from build123d import *

# Parameters (mm, degrees)
F1_DEPTH = 0.43
F2_R     = 0.114538
F2_R_2   = 0.135459
F3_DEPTH = 25
F4_W     = 0.697841
F4_H     = 0.5
F4_W_2   = 0.446198
F4_H_2   = 0.226708
F5_DEPTH = 0.13
F7_DEPTH = 25
F8_W     = 0.044617
F8_H     = 0.11
F8_W_2   = 0.05577
F8_W_3   = 0.03778
F8_W_4   = 0.051917
F9_DEPTH = 0.03


with BuildPart() as f1:
    # F0 (on Top) → F1 (new body)
    with BuildSketch(Plane.XY):
        with BuildLine():
            Line((-17.317478, 8.504073), (-17.317478, 21.504073))
            Line((-17.317478, 21.504073), (-18.245058, 21.504073))
            ThreePointArc((-18.245058, 21.504073), (-18.453947, 21.317083), (-18.662836, 21.504073))
            Line((-18.662836, 21.504073), (-19.242154, 21.504073))
            ThreePointArc((-19.242154, 21.504073), (-19.46455, 21.317806), (-19.686945, 21.504073))
            Line((-19.686945, 21.504073), (-20.317478, 21.504073))
            Line((-20.317478, 21.504073), (-20.317478, 8.504073))
            Line((-20.317478, 8.504073), (-19.500678, 8.504073))
            ThreePointArc((-19.500678, 8.504073), (-19.276541, 8.670717), (-19.052403, 8.504073))
            Line((-19.052403, 8.504073), (-18.489325, 8.504073))
            ThreePointArc((-18.489325, 8.504073), (-18.237854, 8.690502), (-17.986383, 8.504073))
            Line((-17.986383, 8.504073), (-17.317478, 8.504073))
        make_face()
    extrude(amount=F1_DEPTH)

    # F2 (on face) → F3 (cut)
    with BuildSketch(Plane.XY.offset(0.43)):
        with Locations((-17.549288, 8.667056)):
            Circle(F2_R)
        with Locations((-17.561315, 21.304632)):
            Circle(F2_R_2)
    extrude(amount=-F3_DEPTH, mode=Mode.SUBTRACT)

    # F4 (on face) → F5 (join)
    with BuildSketch(Plane.XY.offset(0.43)):
        with Locations((-19.301415, 20.500756)):
            Rectangle(F4_W, F4_H)
        with Locations((-19.301415, 19.600825)):
            Rectangle(F4_W, F4_H)
        with Locations((-19.301415, 18.6384)):
            Rectangle(F4_W, F4_H)
        with Locations((-19.301415, 17.613479)):
            Rectangle(F4_W, F4_H)
        with Locations((-18.021959, 17.250125)):
            Rectangle(F4_W_2, F4_H_2)
        with Locations((-19.301415, 12.958157)):
            Rectangle(F4_W, F4_H)
        with Locations((-19.301415, 11.851003)):
            Rectangle(F4_W, F4_H)
        with Locations((-19.301415, 10.811981)):
            Rectangle(F4_W, F4_H)
        with Locations((-19.301415, 9.670762)):
            Rectangle(F4_W, F4_H)
    extrude(amount=F5_DEPTH)

    # F6 (on face) → F7 (cut)
    with BuildSketch(Plane.XY.offset(0.43)):
        with BuildLine():
            Line((-17.317478, 15.827807), (-17.584291, 15.827807))
            ThreePointArc((-17.584291, 15.827807), (-17.73952, 15.677507), (-17.579334, 15.532503))
            Line((-17.579334, 15.532503), (-17.317478, 15.532503))
            Line((-17.317478, 15.532503), (-17.317478, 15.827807))
        make_face()
    extrude(amount=-F7_DEPTH, mode=Mode.SUBTRACT)

    # F8 (on face) → F9 (join)
    with BuildSketch(Plane.XY.offset(0.43)):
        with Locations((-17.831758, 20.805756)):
            Rectangle(F8_W, F8_H)
        with Locations((-17.837335, 19.574996)):
            Rectangle(F8_W_2, F8_H)
        with Locations((-17.79056, 17.065835)):
            Rectangle(F8_W_3, F8_H)
        with Locations((-17.835408, 10.966537)):
            Rectangle(F8_W_4, F8_H)
    extrude(amount=F9_DEPTH)


solid = f1.part
Part model, mm, in its own coordinate system. Give positions to 0.01 mm unless a question says otherwise; leave off trailing zeros. Loops run counter-clockwise (first coordinate to the right, second up) from the corner with the lowest first, then second, coordinate; pieces in that order, holes last.
(1) Pull direction Y, two halves, no side cores. Call faces 1 (the flat face through (-19, 15, 0)), 2 (the flat face through (-19, 15, 0.43)): pulls with the +Y half, pulls with the -Y half, needs draft (parallel to the pull), parting line crosses it, or undercut.
Return value:
face 1: needs draft
face 2: undercut
(2) Band-saw the part on B-B (x = -19.85). Write the cut outline in (y, z).
Return value:
outline: (8.5, 0) - (21.5, 0) - (21.5, 0.43) - (8.5, 0.43) - close
(3) Drill centre lines: line 1 along Z through (x, y) = (-18.8, 10.75); line 2 along Y through (x, z) = (-18.2, 0.25); line 3 along Y through (x, z) = (-19.6, 0.1). Where is each one in solid material? Low to high.
Return value:
line 1: z = 0 to 0.43
line 2: y = 8.69 to 21.5
line 3: y = 8.5 to 21.36
(4) Band-saw the part on A-A (y = 20.5). Write the cut outline in (x, z), and give its area (3 significant figures).
Return value:
outline: (-20.32, 0) - (-17.32, 0) - (-17.32, 0.43) - (-18.95, 0.43) - (-18.95, 0.56) - (-19.65, 0.56) - (-19.65, 0.43) - (-20.32, 0.43) - close
area: 1.38 mm2
(5) Band-saw the part on C-C (y = 16.5). Write the cut outline in (x, z).
Return value:
outline: (-20.32, 0) - (-17.32, 0) - (-17.32, 0.43) - (-20.32, 0.43) - close
